Part model, mm, in its own coordinate system. Face numbers are marked on the shaded views. A direction names the side the tool comes from. Round coordinates to 2 decimals unless told otherwise and drop trailing zeros. Write each loop counter-clockwise with the first axis right and the second up, starting at its lowest first coordinate (ties: lowest second). Pieces come first, ordered by that corner, then holes. Notation, with made-up numbers: (-24, 52.25) -> (-1, 52.25) arc R19 cw to (-1, 87.25) -> close; hole circle Ø8 at (-4, 71.25). An arc over 180 degrees is marked (long way). Return JSON: item names as keys, results as strings. Group by question number.
(1) Tool access for the marked faces 1 and 2: list every direction of +Z, -Z, +X, -X, +Y, -Y with a clear straight run to the whole face (end or side of a thin tool).
(2) Drop flat-ended pins along their axis: pin 1 Ø4 at (y, z) = (-7.5, -23.5) entering from +X; pin 2 Ø3 at (y, z) = (12.5, -7.5) entering from -X; pin 3 Ø10 at (x, z) = (-9, -27) entering from -Y; pin 4 Ø8.5 at (x, y) = (-2, 1) entering from +Z. Give the stop position or say it passes through.
(3) Saw through at A-A (y = 0). List the corners of the cut face in (x, z), plus the area to 3 significant figures.
(4) Saw through at C-C (y = 12). List the corners of the cut face in (x, z), plus the area to 3 significant figures.
(5) Drill centre lines: L1, parallel to Z at x = 8.5, y = -3.5; L2, parallel to Z at x = 4, y = 12; L3, parallel to X at y = -7, z = -37.5. Where is each one in solid material? Low to high. Write a range as from..to.
(6) Saw through at B-B (z = -31.5). List the corners of the cut face in (x, y).
(7) Mould opens along Y. For the marked faces 3, 4 and 5 say: +Y half, -Y half, draft (parallel to the pull), parting line (faces both ways), or undercut.
(8) Saw through at D-D (y = -11.5). List the corners of the cut face in (x, z).
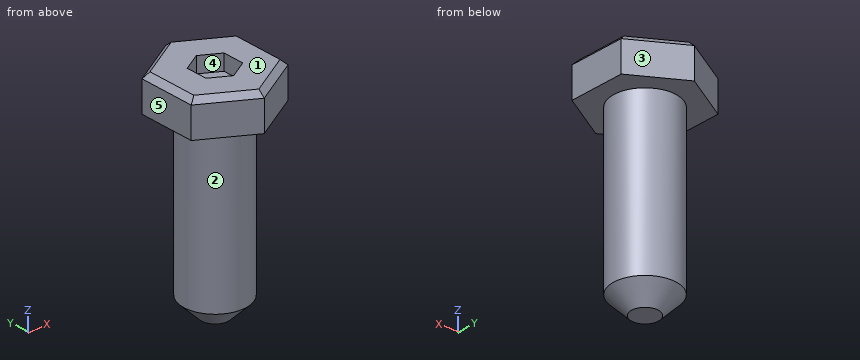
from build123d import *

# Parameters (mm, degrees)
F0_R     = 8.75
F1_DEPTH = 60
F2_DEPTH = 10
F3_SIZE  = 5
F5_DEPTH = 4.4
F6_SIZE  = 1.5


with BuildPart() as f1:
    # F0 (on Top) → F1 (new body)
    with BuildSketch(Plane.XY):
        Circle(F0_R)
    extrude(amount=-F1_DEPTH)

    # F0 (on Top) → F2 (join)
    with BuildSketch(Plane.XY):
        Polygon((13.656054, -7.884326), (13.656054, 7.884326), (0, 15.768653), (-13.656054, 7.884326), (-13.656054, -7.884326), (0, -15.768653), align=None)
        Circle(F0_R, mode=Mode.SUBTRACT)
        Circle(F0_R)
    extrude(amount=-F2_DEPTH)

    # F3
    f3_edges = [f1.edges().sort_by_distance(p)[0] for p in [
        (-8.75, 0, -60),
    ]]
    chamfer(f3_edges, length=F3_SIZE)

    # F4 (on face) → F5 (cut)
    with BuildSketch(Plane.XY):
        Polygon((5.196152, -3), (5.196152, 3), (0, 6), (-5.196152, 3), (-5.196152, -3), (0, -6), align=None)
    extrude(amount=-F5_DEPTH, mode=Mode.SUBTRACT)

    # F6
    f6_edges = [f1.edges().sort_by_distance(p)[0] for p in [
        (-6.828027, -11.826489, 0),
        (6.828027, -11.826489, 0),
        (13.656054, 0, 0),
        (6.828027, 11.826489, 0),
        (-6.828027, 11.826489, 0),
        (-13.656054, 0, 0),
    ]]
    chamfer(f6_edges, length=F6_SIZE)


solid = f1.part
Computed values:
{
 "1": {"face 1": "+Z, +X, -X, +Y, -Y", "face 2": "-Z"},
 "2": {"pin 1": "x = 6.81", "pin 2": "x = -8.26", "pin 3": "y = -7.78", "pin 4": "z = 0"},
 "3": {"outline": "(-13.66, -10) -> (-8.75, -10) -> (-8.75, -55) -> (-3.75, -60) -> (3.75, -60) -> (8.75, -55) -> (8.75, -10) -> (13.66, -10) -> (13.66, -1.5) -> (12.16, 0) -> (5.2, 0) -> (5.2, -4.4) -> (-5.2, -4.4) -> (-5.2, 0) -> (-12.16, 0) -> (-13.66, -1.5) -> close", "area": "1,080 mm2"},
 "4": {"outline": "(-6.53, -10) -> (6.53, -10) -> (6.53, -1.5) -> (3.53, 0) -> (-3.53, 0) -> (-6.53, -1.5) -> close", "area": "126 mm2"},
 "5": {"L1": "-10..0", "L2": "-10..-0.24", "L3": "-5.25..5.25"},
 "6": {"outline": "circle Ø17.5 at (0, 0)"},
 "7": {"face 3": "+Y half", "face 4": "undercut", "face 5": "draft"},
 "8": {"outline": "(-7.39, -10) -> (7.39, -10) -> (7.39, -1.5) -> (4.39, 0) -> (-4.39, 0) -> (-7.39, -1.5) -> close"}
}
